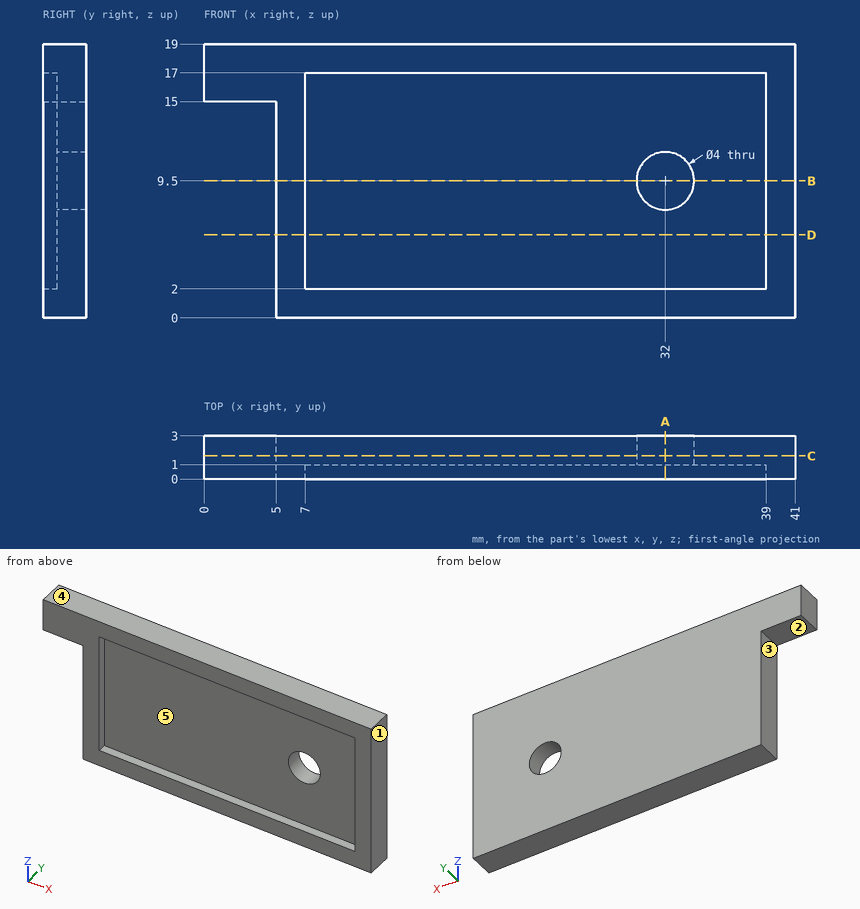
Study the drawing (mm; zero at the part's minimum x, y, z) and answer. A direction names the side the tool comes from. Give positions to 0.01 mm unless a question says otherwise; leave off trailing zeros. Order: outer loops, then holes, each group sorted by start corner. A loop starts at its lowest first (then second) coordinate and runs counter-clockwise, first axis right, second up. Notation, with made-up numbers: (13.25, 58.5) -> (45.25, 58.5) arc R24 ccw to (45.25, 89.5) -> close; hole circle Ø3 at (-34.75, 17.5). An arc over 180 degrees is marked (long way). Write item = value, one per line.
1. Straight lines are drawn through the part: line 1 along Z through (x, y) = (32, 1.9); line 2 along Z through (x, y) = (20.5, 0.25); line 3 along X through (y, z) = (0.25, 7). For each, find the intervals that lie inside material, in ascending order.
Numbers:
line_1 = 0 to 7.5, 11.5 to 19
line_2 = 0 to 2, 17 to 19
line_3 = 5 to 7, 39 to 41
2. A cutting plane is placed at A-A, the plane x = 32. Write down the section's boundary in (y, z).
Numbers:
outline = (0, 0) -> (3, 0) -> (3, 7.5) -> (1, 7.5) -> (1, 2) -> (0, 2) -> close; (0, 17) -> (1, 17) -> (1, 11.5) -> (3, 11.5) -> (3, 19) -> (0, 19) -> close
3. For the marked faces 1 and 2, determine the directions among +Z, -Z, +X, -X, +Y, -Y from which every point of the face is accessible in a straight line to the end or side of a thin tool.
Numbers:
face_1 = +Z, -Z, +X, +Y, -Y
face_2 = -Z, -X, +Y, -Y
4. Given pin 1 (1.5 mm diameter, centred on x = 5.5, z = 13, fed in from -Y); pin 2 (1.5 mm diameter, centred on y = 2, z = 6, fed in from -X); pin 3 (7.5 mm diameter, centred on x = 30.5, z = 10.5, fed in from -Y), each flat-ended and moving along its own axis, determine where each tip first touches the part or whether it passes through.
Numbers:
pin_1 = 0
pin_2 = 5
pin_3 = 1
5. The mould has two halves that part along Z. Classify the marked faces 3, 4 and 5: +Z half, -Z half, draft (parallel to the pull), parting line (faces both ways), or undercut.
Numbers:
face_3 = draft
face_4 = +Z half
face_5 = undercut
6. A cutting plane is placed at D-D, the plane z = 5.75. Write down the section's boundary in (x, y), and give its area (3 significant figures).
Numbers:
outline = (5, 0) -> (7, 0) -> (7, 1) -> (39, 1) -> (39, 0) -> (41, 0) -> (41, 3) -> (5, 3) -> close
area = 76.0 mm²
7. A cutting plane is placed at B-B, the plane z = 9.5. Write down the section's boundary in (x, y).
Numbers:
outline = (5, 0) -> (7, 0) -> (7, 1) -> (30, 1) -> (30, 3) -> (5, 3) -> close; (34, 1) -> (39, 1) -> (39, 0) -> (41, 0) -> (41, 3) -> (34, 3) -> close
8. A cutting plane is placed at C-C, the plane y = 1.6. Write down the section's boundary in (x, z), and give its area (3 significant figures).
Numbers:
outline = (0, 15) -> (5, 15) -> (5, 0) -> (41, 0) -> (41, 19) -> (0, 19) -> close; hole circle Ø4 at (32, 9.5)
area = 691 mm²
